```python
from build123d import *

# Parameters (mm, degrees)
SKETCH_1_R          = 72
SKETCH_1_R_2        = 1.25
EXTRUDE_1_DEPTH     = 5
CUT_EXTRUDE_START   = -10
CUT_EXTRUDE_2_DEPTH = 10
CUT_EXTRUDE_3_DEPTH = 10
EXTRUDE_2_DEPTH     = 5
CUT_EXTRUDE_4_DEPTH = 6
CUT_EXTRUDE_5_DEPTH = 10
FILLET_1_R          = 3
EXTRUDE_3_DEPTH     = 5
SKETCH_13_R         = 1.75
EXTRUDE_4_DEPTH     = 5
FILLET_2_R          = 2
CUT_EXTRUDE_6_DEPTH = 5
FILLET_3_R          = 2


with BuildPart() as part:
    # 草图1 → 凸台-拉伸1 (new body)
    with BuildSketch(Plane.XY):
        Circle(SKETCH_1_R)
        with Locations((25.7, -64)):
            Circle(SKETCH_1_R_2, mode=Mode.SUBTRACT)
        with Locations((25.7, -54)):
            Circle(SKETCH_1_R_2, mode=Mode.SUBTRACT)
        with Locations((25.7, -44)):
            Circle(SKETCH_1_R_2, mode=Mode.SUBTRACT)
        with Locations(Location((-25.7, -44, 0), (0, 0, 180))):
            Circle(SKETCH_1_R_2, mode=Mode.SUBTRACT)
        with Locations(Location((-25.7, -54, 0), (0, 0, 180))):
            Circle(SKETCH_1_R_2, mode=Mode.SUBTRACT)
        with Locations(Location((-25.7, -64, 0), (0, 0, 180))):
            Circle(SKETCH_1_R_2, mode=Mode.SUBTRACT)
        with Locations(Location((-25.255117767, 44.256852877, 0), (0, 0, 180))):
            Circle(SKETCH_1_R_2, mode=Mode.SUBTRACT)
        with Locations(Location((-33.915371804, 49.256852877, 0), (0, 0, 180))):
            Circle(SKETCH_1_R_2, mode=Mode.SUBTRACT)
        with Locations(Location((-42.575625842, 54.256852877, 0), (0, 0, 180))):
            Circle(SKETCH_1_R_2, mode=Mode.SUBTRACT)
        with Locations((-50.955117767, -0.256852877)):
            Circle(SKETCH_1_R_2, mode=Mode.SUBTRACT)
        with Locations((-59.615371804, 4.743147123)):
            Circle(SKETCH_1_R_2, mode=Mode.SUBTRACT)
        with Locations((-68.275625842, 9.743147123)):
            Circle(SKETCH_1_R_2, mode=Mode.SUBTRACT)
        with Locations(Location((50.955117767, -0.256852877, 0), (0, 0, 180))):
            Circle(SKETCH_1_R_2, mode=Mode.SUBTRACT)
        with Locations(Location((59.615371804, 4.743147123, 0), (0, 0, 180))):
            Circle(SKETCH_1_R_2, mode=Mode.SUBTRACT)
        with Locations(Location((68.275625842, 9.743147123, 0), (0, 0, 180))):
            Circle(SKETCH_1_R_2, mode=Mode.SUBTRACT)
        with Locations((25.255117767, 44.256852877)):
            Circle(SKETCH_1_R_2, mode=Mode.SUBTRACT)
        with Locations((33.915371804, 49.256852877)):
            Circle(SKETCH_1_R_2, mode=Mode.SUBTRACT)
        with Locations((42.575625842, 54.256852877)):
            Circle(SKETCH_1_R_2, mode=Mode.SUBTRACT)
    extrude(amount=EXTRUDE_1_DEPTH)

    # 草图3 → 切除-拉伸2 (cut)
    with BuildSketch(Plane.XY.offset(5).offset(CUT_EXTRUDE_START)):
        with BuildLine():
            Line((16.2, -36), (16.2, -70.153830972))
            ThreePointArc((16.2, -70.153830972), (0, -72), (-16.2, -70.153830972))
            Line((-16.2, -70.153830972), (-16.2, -36))
            ThreePointArc((-16.2, -36), (-15.614213562, -34.585786438), (-14.2, -34))
            Line((-14.2, -34), (14.2, -34))
            ThreePointArc((14.2, -34), (15.614213562, -34.585786438), (16.2, -36))
        make_face()
        with BuildLine():
            Line((-23.076914536, 32.029611541), (-52.654999794, 49.106527027))
            ThreePointArc((-52.654999794, 49.106527027), (-62.353829072, 36), (-68.854999794, 21.047303945))
            Line((-68.854999794, 21.047303945), (-39.276914536, 3.970388459))
            ThreePointArc((-39.276914536, 3.970388459), (-37.759276446, 3.770587614), (-36.544863729, 4.702439266))
            Line((-36.544863729, 4.702439266), (-22.344863729, 29.297560734))
            ThreePointArc((-22.344863729, 29.297560734), (-22.145062884, 30.815198824), (-23.076914536, 32.029611541))
        make_face()
        with BuildLine():
            Line((39.276914536, 3.970388459), (68.854999794, 21.047303945))
            ThreePointArc((68.854999794, 21.047303945), (62.353829072, 36), (52.654999794, 49.106527027))
            Line((52.654999794, 49.106527027), (23.076914536, 32.029611541))
            ThreePointArc((23.076914536, 32.029611541), (22.145062884, 30.815198824), (22.344863729, 29.297560734))
            Line((22.344863729, 29.297560734), (36.544863729, 4.702439266))
            ThreePointArc((36.544863729, 4.702439266), (37.759276446, 3.770587614), (39.276914536, 3.970388459))
        make_face()
    extrude(amount=CUT_EXTRUDE_2_DEPTH, mode=Mode.SUBTRACT)

    # 草图5 → 切除-拉伸3 (cut)
    with BuildSketch(Plane.XY.offset(5).offset(CUT_EXTRUDE_START)):
        with BuildLine():
            Line((-41.951694517, 58.515428112), (-6.417930688, 38))
            Line((-6.417930688, 38), (6.417930688, 38))
            Line((6.417930688, 38), (41.951694517, 58.515428112))
            ThreePointArc((41.951694517, 58.515428112), (0, 72), (-41.951694517, 58.515428112))
        make_face()
        with BuildLine():
            Line((71.651694517, 7.073519127), (36.117930688, -13.441908985))
            Line((36.117930688, -13.441908985), (29.7, -24.558091015))
            Line((29.7, -24.558091015), (29.7, -65.58894724))
            ThreePointArc((29.7, -65.58894724), (62.353829072, -36), (71.651694517, 7.073519127))
        make_face()
        with BuildLine():
            Line((-29.7, -65.58894724), (-29.7, -24.558091015))
            Line((-29.7, -24.558091015), (-36.117930688, -13.441908985))
            Line((-36.117930688, -13.441908985), (-71.651694517, 7.073519127))
            ThreePointArc((-71.651694517, 7.073519127), (-62.353829072, -36), (-29.7, -65.58894724))
        make_face()
    extrude(amount=CUT_EXTRUDE_3_DEPTH, mode=Mode.SUBTRACT)

    # 草图6 → 凸台-拉伸2 (add)
    with BuildSketch(Plane.XY.offset(5)):
        Polygon((-71.651694517, 7.073519127), (-29.7, -65.58894724), (-29.7, -55.58894724), (-62.991440479, 2.073519127), align=None)
        Polygon((33.291440479, 53.515428112), (41.951694517, 58.515428112), (-41.951694517, 58.515428112), (-33.291440479, 53.515428112), align=None)
        Polygon((29.7, -55.58894724), (29.7, -65.58894724), (71.651694517, 7.073519127), (62.991440479, 2.073519127), align=None)
    extrude(amount=-EXTRUDE_2_DEPTH)

    # 草图7 → 切除-拉伸4 (cut)
    with BuildSketch(Plane.XY.offset(5)):
        Polygon((-24.883334598, -14.366399928), (-9.827196325, -27), (9.827196325, -27), (24.883334598, -14.366399928), (28.296284065, 4.989398334), (18.46908774, 22.010601666), (0, 28.732799857), (-18.46908774, 22.010601666), (-28.296284065, 4.989398334), align=None)
    extrude(amount=-CUT_EXTRUDE_4_DEPTH, mode=Mode.SUBTRACT)

    # 草图10 → 切除-拉伸5 (cut)
    with BuildSketch(Plane.XY.offset(5).offset(CUT_EXTRUDE_START)):
        with BuildLine():
            Line((-44.842275727, 56.330900114), (-49.923702054, 47.529611541))
            Line((-49.923702054, 47.529611541), (-52.654999794, 49.106527027))
            ThreePointArc((-52.654999794, 49.106527027), (-48.882282835, 52.863242663), (-44.842275727, 56.330900114))
        make_face()
        with BuildLine():
            Line((-68.854999794, 21.047303945), (-66.123702054, 19.470388459))
            Line((-66.123702054, 19.470388459), (-71.20512838, 10.669099886))
            ThreePointArc((-71.20512838, 10.669099886), (-70.22205249, 15.901677398), (-68.854999794, 21.047303945))
        make_face()
        with BuildLine():
            Line((52.654999794, 49.106527027), (49.923702054, 47.529611541))
            Line((49.923702054, 47.529611541), (44.842275727, 56.330900114))
            ThreePointArc((44.842275727, 56.330900114), (48.882282835, 52.863242663), (52.654999794, 49.106527027))
        make_face()
        with BuildLine():
            Line((66.123702054, 19.470388459), (68.854999794, 21.047303945))
            ThreePointArc((68.854999794, 21.047303945), (70.22205249, 15.901677398), (71.20512838, 10.669099886))
            Line((71.20512838, 10.669099886), (66.123702054, 19.470388459))
        make_face()
        with BuildLine():
            Line((16.2, -70.153830972), (16.2, -67))
            Line((16.2, -67), (26.362852653, -67))
            ThreePointArc((26.362852653, -67), (21.339769655, -68.764920061), (16.2, -70.153830972))
        make_face()
        with BuildLine():
            Line((-16.2, -67), (-16.2, -70.153830972))
            ThreePointArc((-16.2, -70.153830972), (-21.339769655, -68.764920061), (-26.362852653, -67))
            Line((-26.362852653, -67), (-16.2, -67))
        make_face()
    extrude(amount=CUT_EXTRUDE_5_DEPTH, mode=Mode.SUBTRACT)

    # 圆角1
    fillet_1_edges = [part.edges().sort_by_distance(p)[0] for p in [
        (16.2, -67, 2.5),
        (-16.2, -67, 2.5),
        (-66.123702054, 19.470388459, 2.5),
        (-49.923702054, 47.529611541, 2.5),
        (49.923702054, 47.529611541, 2.5),
        (66.123702054, 19.470388459, 2.5),
    ]]
    fillet(fillet_1_edges, radius=FILLET_1_R)

    # 草图12 → 凸台-拉伸3 (add)
    with BuildSketch(Plane(origin=(0, 0, 0), x_dir=(-1, 0, 0), z_dir=(0, 0, -1))):
        Polygon((-29.7, -24.558091015), (-29.7, -55.58894724), (-62.991440479, 2.073519127), (-36.117930688, -13.441908985), align=None)
    extrude(amount=-EXTRUDE_3_DEPTH)

    # 草图13 → 凸台-拉伸4 (add)
    with BuildSketch(Plane(origin=(50.675847258, -29.257714056, 0), x_dir=(0, 0, -1), z_dir=(0.8660254037844392, -0.49999999999999906, 0))):
        Polygon((0, 21), (10.656854249, 21), (14, 17.656854249), (14, 12.966018868), (7, 1.766018868), (7, -1.766018868), (14, -12.966018868), (14, -17.656854249), (10.656854249, -21), (0, -21), align=None)
        with Locations(Location((5, 8, 0), (0, 0, 90))):
            Circle(SKETCH_13_R, mode=Mode.SUBTRACT)
        with Locations(Location((10, 16, 0), (0, 0, 90))):
            Circle(SKETCH_13_R, mode=Mode.SUBTRACT)
        with Locations(Location((5, -8, 0), (0, 0, 270))):
            Circle(SKETCH_13_R, mode=Mode.SUBTRACT)
        with Locations(Location((10, -16, 0), (0, 0, 270))):
            Circle(SKETCH_13_R, mode=Mode.SUBTRACT)
    extrude(amount=-EXTRUDE_4_DEPTH)

    # 圆角2
    fillet_2_edges = [part.edges().sort_by_distance(p)[0] for p in [
        (46.34572024, -26.757714056, 0),
        (38.010783749, -46.194247536, 0),
        (59.010783749, -9.821180577, 0),
    ]]
    fillet(fillet_2_edges, radius=FILLET_2_R)

    # 草图14 → 切除-拉伸6 (cut)
    with BuildSketch(Plane(origin=(0, 0, 0), x_dir=(-1, 0, 0), z_dir=(0, 0, -1))):
        with BuildLine():
            Line((-29.7, -24.826040208), (-29.7, -40.826040208))
            ThreePointArc((-29.7, -40.826040208), (-30.441180955, -41.791966034), (-31.566025404, -41.326040208))
            Line((-31.566025404, -41.326040208), (-51.57241336, -6.673959792))
            ThreePointArc((-51.57241336, -6.673959792), (-51.413494737, -5.466853011), (-50.206387956, -5.307934389))
            Line((-50.206387956, -5.307934389), (-36.349981495, -13.307934389))
            ThreePointArc((-36.349981495, -13.307934389), (-36.142874714, -13.466853011), (-35.983956091, -13.673959792))
            Line((-35.983956091, -13.673959792), (-29.833974596, -24.326040208))
            ThreePointArc((-29.833974596, -24.326040208), (-29.734074174, -24.567221163), (-29.7, -24.826040208))
        make_face()
    extrude(amount=-CUT_EXTRUDE_6_DEPTH, mode=Mode.SUBTRACT)

    # 圆角3
    fillet_3_edges = [part.edges().sort_by_distance(p)[0] for p in [
        (6.417930688, 38, 2.5),
        (-6.417930688, 38, 2.5),
        (-36.117930688, -13.441908985, 2.5),
        (-29.7, -24.558091015, 2.5),
        (-62.991440479, 2.073519127, 2.5),
        (-29.7, -55.58894724, 2.5),
        (33.291440479, 53.515428112, 2.5),
        (-33.291440479, 53.515428112, 2.5),
    ]]
    fillet(fillet_3_edges, radius=FILLET_3_R)


solid = part.part
```
The listing builds one solid part. Answer for the finished solid, in the listing's coordinates (mm). A direction names the side the tool comes from. Round coordinates to 2 decimals unless told otherwise and drop trailing zeros. Order: outer loops, then holes, each group sorted by start corner. A loop starts at its lowest first (then second) coordinate and runs counter-clockwise, first axis right, second up. Notation, with made-up numbers: (13, -3.5) -> (39, -3.5) arc R21 ccw to (39, 33.5) -> close; hole circle Ø10 at (-22, 2.5). An arc over 180 degrees is marked (long way). Answer as CSV lines item,"result". Start each with the question number.
(1) A tool of negligible diameter and unlimited length cuts with its end or side. For faces 1 (the face through (40.655, -41.684, -11.735)), 2 (the face through (38.04, -46.21, -6.39)), 3 (the face through (-32.87, -19.07, 2.46)), from which of +Z, -Z, +X, -X, +Y, -Y can it reach the whole face along a straight path? Write none if from no direction.
(2) The part is cut by section D-D (z = 2.5). Count the separate pieces of the cut face and the enclosed holes in it, then the cut area to 3 significant figures.
(3) Flat-ended cylindrical pins translate along their axes: pin 1 Ø3 at (x, z) = (-17, -2.5) entering from +Y; pin 2 Ø1.7 at (x, y) = (50, -27.5) entering from -Z; pin 3 Ø6 at (x, y) = (15, -43) entering from -Z; pin 4 Ø5.5 at (y, z) = (-47, 3) entering from +X. Find the tip coordinate at first contact, or state that the pin passes through.
(4) For a pull along Y with two mould halves and no side action, classify faces 4 (the face through (46.493, -26.503, -6.751)), 5 (the face through (0, 53.515, 3)), 6 (the face through (-17.1, -66.14, 2.54)) as +Y half, -Y half, draft (parallel to the pull), parting line (faces both ways), or undercut.
(5) The part is cut by section C-C (x = 2.5). Determine the outline of the cut face in (y, z), then the cut area to 3 significant figures.
(6) The part is cut by section A-A (x = -12). Determine the outline of the cut face in (y, z).
(7) Find the intervals of material crossed by probe 1 along X at (y, z) = (18, 2); probe 2 along Y at (x, z) = (-31, 3); probe 3 along X at (y, z) = (-9.5, 1.75), in increasing order. Write a range as from..to.
(8) The part is cut by section B-B (y = 40.5). Determine the outline of the cut face in (x, z), then the cut area to 3 significant figures.
Evaluation:
1,face 1,"none"
1,face 2,"-Z, -X, -Y"
1,face 3,"+Z, -Z"
2,separate pieces,"1"
2,enclosed holes,"22"
2,area,"6,270 mm²"
3,pin 1,"through"
3,pin 2,"z = -7.17"
3,pin 3,"z = 0"
3,pin 4,"x = 42.02"
4,face 4,"+Y half"
4,face 5,"undercut"
4,face 6,"-Y half"
5,outline,"(-34, 0) -> (-27, 0) -> (-27, 5) -> (-34, 5) -> close; (27.82, 0) -> (38, 0) -> (38, 5) -> (27.82, 5) -> close; (53.52, 0) -> (58.52, 0) -> (58.52, 5) -> (53.52, 5) -> close"
5,area,"111 mm²"
6,outline,"(-34, 0) -> (-25.18, 0) -> (-25.18, 5) -> (-34, 5) -> close; (24.37, 0) -> (41.22, 0) -> (41.22, 5) -> (24.37, 5) -> close; (53.52, 0) -> (58.52, 0) -> (58.52, 5) -> (53.52, 5) -> close"
7,probe 1,"-66.47..-63.58, -28.87..-20.78, 20.78..28.87, 63.58..66.47"
7,probe 2,"-63.34..-50, -22.31..14.31, 36.6..58.52"
7,probe 3,"-62.08..-56.31, -42.95..-25.74, 25.74..42.95, 49.94..62.08"
8,outline,"(-37.75, 0) -> (-10.75, 0) -> (-10.75, 5) -> (-37.75, 5) -> close; (10.75, 0) -> (37.75, 0) -> (37.75, 5) -> (10.75, 5) -> close"
8,area,"270 mm²"
